Solid Edge part; units mm, degrees
sketch "Sketch1" plane through (0, 0, 0) normal (0, 0, 1) x (1, 0, 0)
  circle A0 centre (0, 0) radius 5
extrude "Protrusion1" add sketch "Sketch1" along normal blind 6
sketch "Sketch2" plane through (0, 0, 6) normal (0, 0, 1) x (0, 1, 0)
  line L0 (0, 2.8868) -> (2.5, 1.4434)
  line L1 (2.5, 1.4434) -> (2.5, -1.4434)
  line L2 (2.5, -1.4434) -> (0, -2.8868)
  line L3 (0, -2.8868) -> (-2.5, -1.4434)
  line L4 (-2.5, -1.4434) -> (-2.5, 1.4434)
  line L5 (-2.5, 1.4434) -> (0, 2.8868)
extrude "Cutout1" cut sketch "Sketch2" against normal blind 3
fillet "Round1" radius 0.6 1 edges at (-5, 0, 6)
sketch "Sketch3" plane through (0, 0, 0) normal (1, 0, 0) x (0, 1, 0)
  line L0 (-2.3865, -16) -> (0, -16)
  line L1 (-3, -15.3865) -> (-2.3865, -16)
  line L2 (-3, -3) -> (-3, -15.3865)
  line L3 (-2.3865, -3) -> (-3, -3)
  line L4 (-2.3865, -2.99) -> (-2.3865, -3)
  line L5 (-3, -2.99) -> (-2.3865, -2.99)
  line L6 (-3, -0.25) -> (-3, -2.99)
  arc A0 (-3, -0.25) -> (-3.25, 0) centre (-3.25, -0.25) ccw
revolve "RevolvedProtrusion1" add sketch "Sketch3" angle 360 about axis through (0, 0, -60.325) along (0, 0, 1) material side at (0, -1.1932, -15.95)
cosmetic_thread "Thread1"
sketch "Sketch4" plane through (0, 0, 0) normal (0, -1, 0) x (1, 0, 0)
  line L0 (-2.86, 6) -> (0, 4.3488)
revolve "RevolvedCutout1" cut sketch "Sketch4" angle 360 about axis through (0, 0, 57.15) along (0, 0, -1) material side at (-1.405, 0, 5.2177)
properties material "Steel"
CAD build for the part. Positions are in the model's coordinates, mm. A direction names the side the tool comes from. Give positions to 0.01 mm unless a question says otherwise; leave off trailing zeros. Loops run counter-clockwise (first coordinate to the right, second up) from the corner with the lowest first, then second, coordinate; pieces in that order, holes last. Notation, with made-up numbers: (45, 83.5) - (83, 83.5) arc R24 ccw to (83, 111.5) - close; hole circle Ø9 at (-24, -1). An arc over 180 degrees is marked (long way). Put each result on its own line as item: value.
Q1. Slice it at C-C (z = -14). Give the cut face in (x, y), plus the area to 3 significant figures.
Filled in:
outline: circle Ø6 at (0, 0)
area: 28.3 mm²
Q2. Tool access for faces 1 (the face through (1, -3, 6)), 2 (the face through (2.297, 1.305, 5.874)), 3 (the face through (3.3, -1, 0)): list every direction of +Z, -Z, +X, -X, +Y, -Y with a clear straight run to the whole face (end or side of a thin tool).
Filled in:
face 1: +Z, +X, -X, +Y, -Y
face 2: +Z
face 3: -Z
Q3. Probe line 1 along Z through (x, y) = (4.25, 1); line 2 along Y through (x, z) = (-4, 3.75); line 3 along Y through (x, z) = (-1.5, 3.25). List the from-to ranges inside material, lowest first.
Filled in:
line 1: z = 0 to 6
line 2: y = -3 to 3
line 3: y = -4.77 to -2.4, 2.4 to 4.77
Q4. Flat gauge pins, fed straight in: pin 1 (5 mm diameter, centred on x = 0.5, z = -12, fed in from -Y); pin 2 (1.5 mm diameter, centred on y = -1.5, z = -12, fed in from +X); pin 3 (2.5 mm diameter, centred on x = 0, y = 1, fed in from +Z). Where does each tip first touch, or does it go through?
Filled in:
pin 1: stops at y = -3
pin 2: stops at x = 2.9
pin 3: stops at z = 3
Q5. Slice it at B-B (z = 1). Give the cut face in (x, y), plus the area to 3 significant figures.
Filled in:
outline: circle Ø10 at (0, 0)
area: 78.5 mm²
